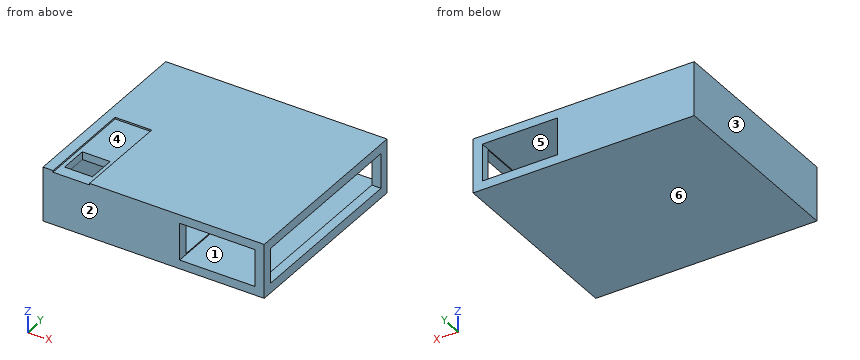
```python
from build123d import *

# Parameters (mm, degrees)
F0_W     = 63.503295
F0_H     = 55.21382
F1_DEPTH = 15.6
F2_W     = 21.611847
F2_H     = 10.657895
F3_DEPTH = 60.6
F4_W     = 49.736842
F4_H     = 10.06579
F5_DEPTH = 59.6
F6_W     = 8
F6_H     = 8
F7_DEPTH = 6.1
F8_W     = 10.503809
F8_H     = 0.480202
F9_DEPTH = 27.9


with BuildPart() as f1:
    # F0 (on Top) → F1 (new body)
    with BuildSketch(Plane.XY):
        with Locations((31.751647, 27.60691)):
            Rectangle(F0_W, F0_H)
    extrude(amount=F1_DEPTH)

    # F2 (on face) → F3 (cut)
    with BuildSketch(Plane.XZ):
        with Locations((50.032899, 7.845395)):
            Rectangle(F2_W, F2_H)
    extrude(amount=-F3_DEPTH, mode=Mode.SUBTRACT)

    # F4 (on face) → F5 (cut)
    with BuildSketch(Plane.YZ.offset(63.503295)):
        with Locations((27.680923, 7.845395)):
            Rectangle(F4_W, F4_H)
    extrude(amount=-F5_DEPTH, mode=Mode.SUBTRACT)

    # F6 (on face) → F7 (cut)
    with BuildSketch(Plane.XY.offset(15.6)):
        with Locations((8, 7.41359)):
            Rectangle(F6_W, F6_H)
    extrude(amount=-F7_DEPTH, mode=Mode.SUBTRACT)

    # F8 (on face) → F9 (cut)
    with BuildSketch(Plane.XZ):
        with Locations((8.121265, 15.359899)):
            Rectangle(F8_W, F8_H)
    extrude(amount=-F9_DEPTH, mode=Mode.SUBTRACT)


solid = f1.part
```
Can you work these out from the model? Positions are in its coordinate system, mm. Face numbers are marked on the shaded views. A direction names the side the tool comes from. Round coordinates to 2 decimals unless told otherwise and drop trailing zeros. Loops run counter-clockwise (first coordinate to the right, second up) from the corner with the lowest first, then second, coordinate; pieces in that order, holes last. Notation, with made-up numbers: (13, 22.25) -> (60, 22.25) arc R21 cw to (60, 49.25) -> close; hole circle Ø2 at (54.5, 4). An arc over 180 degrees is marked (long way). One line per item, written item: value. Start each with the question number.
1. If we section it at C-C, the plane x = 37: Write out the boundary of the cut face in (y, z), then the cut area to 3 significant figures.
2. If we mould it in two halves opening along X, with no side actions, what happens to the marked faces 3, 4, 5 and 6? For each: pulls with the +X half, pulls with the -X half, needs draft (parallel to the pull), parting line crosses it, or undercut.
3. If we section it at D-D, the plane y = 15.5: Write out the boundary of the cut face in (x, z), then the cut area to 3 significant figures.
4. If I drill on probe 1 along Z at (x, y) = (33, 51.5); probe 2 along Y at (x, z) = (26, 8.25); probe 3 along Z at (x, y) = (7.5, 15), over which ranges is the centre line in solid material (lowest first)?
5. For the marked faces 1 and 2, which set-ups out of +Z, -Z, +X, -X, +Y, -Y let a thin tool reach every point of the face, with its end or its side?
6. If we section it at B-B, the plane z = 11.5: Write out the boundary of the cut face in (x, y), then the cut area to 3 significant figures.
7. For pin 1 (3 mm diameter, centred on y = 18, z = 8.5, fed in from +X), with a flat end and sliding along its axis, tell me the tip position at first contact or that it passes through.
8. If we section it at A-A, the plane x = 54: Write out the boundary of the cut face in (y, z), then the cut area to 3 significant figures.
Calculated:
1. outline: (0, 0) -> (55.21, 0) -> (55.21, 15.6) -> (0, 15.6) -> close; hole (2.81, 2.81) -> (52.55, 2.81) -> (52.55, 12.88) -> (2.81, 12.88) -> close
1. area: 361 mm²
2. face 3: pulls with the -X half
2. face 4: undercut
2. face 5: undercut
2. face 6: needs draft
3. outline: (0, 0) -> (63.5, 0) -> (63.5, 2.81) -> (60.84, 2.81) -> (60.84, 2.52) -> (39.23, 2.52) -> (39.23, 2.81) -> (3.9, 2.81) -> (3.9, 12.88) -> (39.23, 12.88) -> (39.23, 13.17) -> (60.84, 13.17) -> (60.84, 12.88) -> (63.5, 12.88) -> (63.5, 15.6) -> (13.37, 15.6) -> (13.37, 15.12) -> (2.87, 15.12) -> (2.87, 15.6) -> (0, 15.6) -> close
3. area: 373 mm²
4. probe 1: z = 0 to 2.81, 12.88 to 15.6
4. probe 2: y = 0 to 2.81, 52.55 to 55.21
4. probe 3: z = 0 to 2.81, 12.88 to 15.12
5. face 1: +Y, -Y
5. face 2: +Z, -Z, +X, -X, -Y
6. outline: (0, 0) -> (39.23, 0) -> (39.23, 2.81) -> (3.9, 2.81) -> (3.9, 52.55) -> (39.23, 52.55) -> (39.23, 55.21) -> (0, 55.21) -> close; (60.84, 0) -> (63.5, 0) -> (63.5, 2.81) -> (60.84, 2.81) -> close; (60.84, 52.55) -> (63.5, 52.55) -> (63.5, 55.21) -> (60.84, 55.21) -> close
6. area: 424 mm²
7. pin 1: stops at x = 3.9
8. outline: (0, 0) -> (55.21, 0) -> (55.21, 2.52) -> (0, 2.52) -> close; (0, 13.17) -> (55.21, 13.17) -> (55.21, 15.6) -> (0, 15.6) -> close
8. area: 273 mm²
